Check sheet for the modelled part. Datum: model origin and axes. Units: mm. Round coordinates to 2 decimals unless told otherwise and drop trailing zeros. Write each loop counter-clockwise with the first axis right and the second up, starting at its lowest first coordinate (ties: lowest second). Pieces come first, ordered by that corner, then holes.
Item 1: Depth check by flat-ended pin: pin 1 (1 mm diameter, centred on x = -3, z = 1.5, fed in from -Y); pin 2 (1 mm diameter, centred on x = 1.5, z = 0.5, fed in from +Y). Enter the tip coordinate at first touch or a pass-through.
Item 2: Section check A-A, the plane x = 0. Record the cut outline in (y, z).
Item 3: Release check for a two-part mould opening along Y. For faces 1 (the cylindrical face through (-0.208, 16.586, 0.986)), 2 (the cylindrical face through (0.16, 22.5, 0.99)), 3 (the flat face through (7.5, 8, 1)) record: pulls with the +Y half, pulls with the -Y half, needs draft (parallel to the pull), parting line crosses it, or undercut.
Item 4: Section check B-B, the plane z = 0.4. Record the cut outline in (x, y).
Item 5: Section check D-D, the plane y = 19.5. Record the cut outline in (x, z), plus the area to 3 significant figures.
Item 6: Material ranges on line 1 along Y through (x, z) = (0, 0.65); line 2 along Y through (x, z) = (-1.25, 1.25); line 3 along X through (y, z) = (14.75, 1), recorded low to high.
Item 7: Section check C-C, the plane x = 4.5. Record the cut outline in (y, z).
from build123d import *

# Parameters (mm, degrees)
SKETCH_R     = 1.6
SKETCH_R_2   = 2
PAD_DEPTH    = 2
CHAMFER_SIZE = 1


with BuildPart() as part:
    # Sketch → Pad (new body)
    with BuildSketch(Plane.XY):
        with BuildLine():
            ThreePointArc((7.5, 15), (0, 22.5), (-7.5, 15))
            Line((-7.5, 15), (-7.5, 0))
            ThreePointArc((-7.5, 0), (0, -7.5), (7.5, 0))
            Line((7.5, 15), (7.5, 0))
        make_face()
        with Locations((0, 15)):
            Circle(SKETCH_R, mode=Mode.SUBTRACT)
        Circle(SKETCH_R_2, mode=Mode.SUBTRACT)
    extrude(amount=PAD_DEPTH)

    # Chamfer
    chamfer_edges = [part.edges().sort_by_distance(p)[0] for p in [
        (-2, 0, 2),
    ]]
    chamfer(chamfer_edges, length=CHAMFER_SIZE)


solid = part.part
Values found:
1. pin 1: stops at y = -7.07
1. pin 2: stops at y = 22.43
2. outline: (-7.5, 0) - (-2, 0) - (-2, 1) - (-3, 2) - (-7.5, 2) - close; (2, 0) - (13.4, 0) - (13.4, 2) - (3, 2) - (2, 1) - close; (16.6, 0) - (22.5, 0) - (22.5, 2) - (16.6, 2) - close
3. face 1: undercut
3. face 2: pulls with the +Y half
3. face 3: needs draft
4. outline: (-7.5, 0) arc R7.5 ccw to (7.5, 0) - (7.5, 15) arc R7.5 ccw to (-7.5, 15) - close; hole circle Ø4 at (0, 0); hole circle Ø3.2 at (0, 15)
5. outline: (-6, 0) - (6, 0) - (6, 2) - (-6, 2) - close
5. area: 24.0 mm2
6. line 1: y = -7.5 to -2, 2 to 13.4, 16.6 to 22.5
6. line 2: y = -7.4 to -1.87, 1.87 to 14, 16 to 22.4
6. line 3: x = -7.5 to -1.58, 1.58 to 7.5
7. outline: (-6, 0) - (21, 0) - (21, 2) - (-6, 2) - close
